Read the model definition and answer for the solid it produces. Units are mm, in the model's axes. Give positions to 0.01 mm unless a question says otherwise; leave off trailing zeros. Order: outer loops, then holes, each group sorted by start corner. A loop starts at its lowest first (then second) coordinate and runs counter-clockwise, first axis right, second up. Notation, with made-up numbers: (4.25, -37) -> (43.25, -37) arc R33 cw to (43.25, -6) -> close; hole circle Ø4 at (-6, -36). An arc over 180 degrees is marked (long way). Use one line per item in the form item = value.
```python
from build123d import *

# Parameters (mm, degrees)
PAD_DEPTH    = 13.5
PAD001_DEPTH = 1
PAD008_DEPTH = 1


with BuildPart() as part:
    # Sketch → Pad (new body)
    with BuildSketch(Plane.YZ):
        with BuildLine():
            Line((-8, 0), (-8, -8))
            Line((-8, -8), (8, -8))
            Line((8, 0), (8, -8))
            Line((8, 0), (6.1, 0))
            ThreePointArc((-6.1, 0), (0, -6.1), (6.1, 0))
            ThreePointArc((-4.3133513652, 4.3133513652), (-5.6356651483, 2.3343689374), (-6.1, 0))
            Line((-5.6568542495, 5.6568542495), (-4.3133513652, 4.3133513652))
            ThreePointArc((-5.6568542495, 5.6568542495), (-7.3910362601, 3.0614674589), (-8, 0))
        make_face()
    extrude(amount=PAD_DEPTH)

    # Sketch001 → Pad001 (join)
    with BuildSketch(Plane.YZ):
        with BuildLine():
            ThreePointArc((-4.1012193309, 4.1012193309), (-2.2195639077, -5.3585012886), (5.8, 0))
            Line((5.8, 0), (6.1, 0))
            ThreePointArc((-4.3133513652, 4.3133513652), (-2.3343689374, -5.6356651483), (6.1, 0))
            Line((-4.1012193309, 4.1012193309), (-4.3133513652, 4.3133513652))
        make_face()
    extrude(amount=PAD001_DEPTH)

    # Sketch013 (on Face5 of Pad001) → Pad008 (join)
    with BuildSketch(Plane.YZ.offset(13.5)):
        with BuildLine():
            ThreePointArc((-4.3133513652, 4.3133513652), (-2.3343689374, -5.6356651483), (6.1, 0))
            Line((5.8, 0), (6.1, 0))
            ThreePointArc((-4.1012193309, 4.1012193309), (-2.2195639077, -5.3585012886), (5.8, 0))
            Line((-4.3133513652, 4.3133513652), (-4.1012193309, 4.1012193309))
        make_face()
    extrude(amount=-PAD008_DEPTH)


solid = part.part
```
Item 1: The part is cut by section D-D on z = 0.5. Give the vertices of the cut face in (x, y).
Checks:
outline = (0, -7.98) -> (13.5, -7.98) -> (13.5, -5.78) -> (12.5, -5.78) -> (12.5, -6.08) -> (1, -6.08) -> (1, -5.78) -> (0, -5.78) -> close
Item 2: Straight lines are drawn through the part: L1, parallel to Y at x = 9, z = -1.5; L2, parallel to Z at x = 13.3, y = 0; L3, parallel to Z at x = 7.5, y = -4.75. For each, find the intervals that lie inside material, in ascending order. Write a range as from..to.
Checks:
L1 = -8..-5.91, 5.91..8
L2 = -8..-5.8
L3 = -8..-3.83, 3.83..4.75
Item 3: Determine the mould class of faces 1 (the cylindrical face through (0.493, -2.366, -5.295)), 2 (the flat face through (7, 7, 0)), 3 (the flat face through (13.5, -2, -6)) for opening direction Z: +Z half, -Z half, draft (parallel to the pull), parting line (faces both ways), or undercut.
Checks:
face_1 = undercut
face_2 = +Z half
face_3 = draft
Item 4: The part is cut by section C-C on x = 3. Give the vertices of the cut face in (y, z), and give its area (3 significant figures).
Checks:
outline = (-8, -8) -> (8, -8) -> (8, 0) -> (6.1, 0) arc R6.1 cw (long way) to (-4.31, 4.31) -> (-5.66, 5.66) arc R8 ccw to (-8, 0) -> close
area = 80.1 mm²
Item 5: Given pin 1 Ø3 at (x, y) = (9, 2.5) entering from +Z; pin 2 Ø3 at (x, y) = (2, -0.5) entering from +Z; pin 3 Ø1.1 at (x, y) = (5.5, 7) entering from +Z, each flat-ended and moving along its own axis, determine where each tip first touches the part or whether it passes through.
Checks:
pin_1 = -4.61
pin_2 = -5.57
pin_3 = 0
Item 6: The part is cut by section A-A on z = -2. Give the vertices of the cut face in (x, y).
Checks:
outline = (0, -8) -> (13.5, -8) -> (13.5, -5.44) -> (12.5, -5.44) -> (12.5, -5.76) -> (1, -5.76) -> (1, -5.44) -> (0, -5.44) -> close; (0, 5.44) -> (1, 5.44) -> (1, 5.76) -> (12.5, 5.76) -> (12.5, 5.44) -> (13.5, 5.44) -> (13.5, 8) -> (0, 8) -> close
Item 7: The part is cut by section B-B on y = 0. Give the vertices of the cut face in (x, z).
Checks:
outline = (0, -8) -> (13.5, -8) -> (13.5, -5.8) -> (12.5, -5.8) -> (12.5, -6.1) -> (1, -6.1) -> (1, -5.8) -> (0, -5.8) -> close
